Could you check a few things on this drawing? It's one solid part, dimensions in mm from its lowest x, y, z. Coordinates: 2 decimals unless noted, no trailing zeros. Order: outer loops, then holes, each group sorted by start corner. A loop starts at its lowest first (then second) coordinate and runs counter-clockwise, first axis right, second up. Notation, with made-up numbers: (-16.5, 27.25) -> (32.5, 27.25) arc R13 cw to (32.5, 34.25) -> close; hole circle Ø1 at (-11.75, -1). An arc over 180 degrees is marked (long way). Answer as CSV lines item,"result".
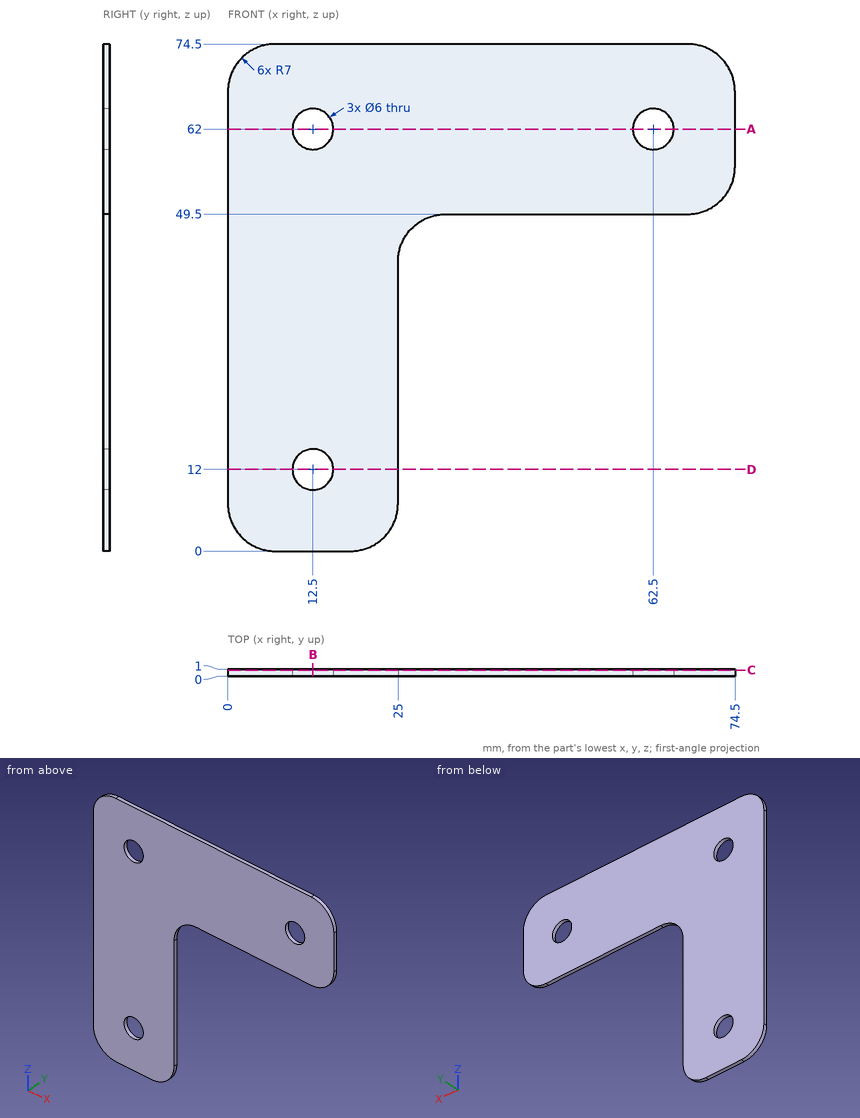
Q1. Imagine slicing it at A-A (z = 62). List the corners of the cut face in (x, y) for me, and give its area (3 significant figures).
Solution:
outline,"(0, 0) -> (9.5, 0) -> (9.5, 1) -> (0, 1) -> close; (15.5, 0) -> (59.5, 0) -> (59.5, 1) -> (15.5, 1) -> close; (65.5, 0) -> (74.5, 0) -> (74.5, 1) -> (65.5, 1) -> close"
area,"62.5 mm2"
Q2. Imagine slicing it at B-B (x = 12.5). List the corners of the cut face in (y, z) for me.
Solution:
outline,"(0, 0) -> (1, 0) -> (1, 9) -> (0, 9) -> close; (0, 15) -> (1, 15) -> (1, 59) -> (0, 59) -> close; (0, 65) -> (1, 65) -> (1, 74.5) -> (0, 74.5) -> close"
Q3. If I drill on line 1 (Z direction, x = 12.5, y = 0.5); line 2 (X direction, y = 0.35, z = 62); line 3 (X direction, y = 0.85, z = 68), over which ranges is the centre line in solid material (lowest first)?
Solution:
line 1,"0 to 9, 15 to 59, 65 to 74.5"
line 2,"0 to 9.5, 15.5 to 59.5, 65.5 to 74.5"
line 3,"0.02 to 74.48"
Q4. Imagine slicing it at C-C (y = 0.85). List the corners of the cut face in (x, z) for me, and give its area (3 significant figures).
Solution:
outline,"(0, 7) arc R7 ccw to (7, 0) -> (18, 0) arc R7 ccw to (25, 7) -> (25, 42.5) arc R7 cw to (32, 49.5) -> (67.5, 49.5) arc R7 ccw to (74.5, 56.5) -> (74.5, 67.5) arc R7 ccw to (67.5, 74.5) -> (7, 74.5) arc R7 ccw to (0, 67.5) -> close; hole circle Ø6 at (12.5, 12); hole circle Ø6 at (12.5, 62); hole circle Ø6 at (62.5, 62)"
area,"2,970 mm2"
Q5. Imagine slicing it at D-D (z = 12). List the corners of the cut face in (x, y) for me, and give its area (3 significant figures).
Solution:
outline,"(0, 0) -> (9.5, 0) -> (9.5, 1) -> (0, 1) -> close; (15.5, 0) -> (25, 0) -> (25, 1) -> (15.5, 1) -> close"
area,"19.0 mm2"
